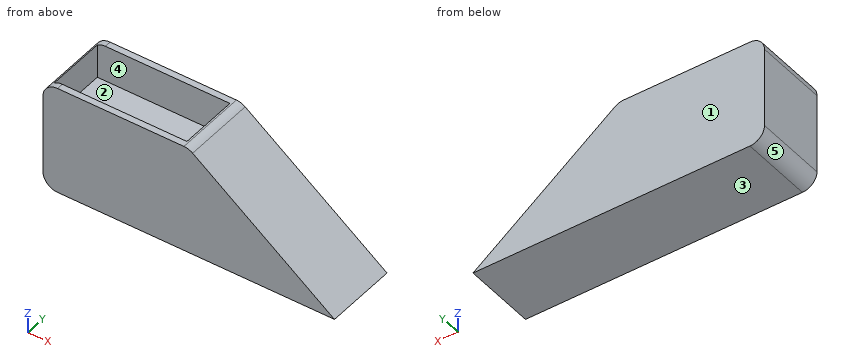
```python
from build123d import *

# Parameters (mm, degrees)
F1_DEPTH    = 25.4
F2_W        = 46.228
F2_H        = 20.828
F3_DEPTH    = 12.7
F4_T1_DEPTH = 50.8
F4_T3_DEPTH = 33.8666666667


# Not quite as in the source:
# - a fillet or chamfer that OpenCascade refuses, or shapes differently, is made with other operations: its cross-section is extruded or revolved along the edge and cut away or added


with BuildPart() as f1:
    # F0 (on Front) → F1 (new body)
    with BuildSketch(Plane.XZ):
        Polygon((0, 38.1), (0, 0), (101.6, 0), (50.8, 38.1), align=None)
    extrude(amount=F1_DEPTH)

    # F2 (on face) → F3 (cut)
    with BuildSketch(Plane.XY.offset(38.1)):
        with Locations((25.4, -12.7)):
            Rectangle(F2_W, F2_H)
    extrude(amount=-F3_DEPTH, mode=Mode.SUBTRACT)

    # F4: fillet of radius 5.08 on 3 edges, made by hand

    # F4_s2 → F4_t1 (cut)
    with BuildSketch(Plane.XZ.offset(-12.7)):
        with BuildLine():
            ThreePointArc((0, 33.02), (1.4878975516, 36.6121024484), (5.08, 38.1))
            Line((5.08, 38.1), (0, 38.1))
            Line((0, 38.1), (0, 33.02))
        make_face()
        with BuildLine():
            ThreePointArc((0, 5.08), (1.4878975516, 1.4878975516), (5.08, 0))
            Line((5.08, 0), (0, 0))
            Line((0, 0), (0, 5.08))
        make_face()
    extrude(amount=F4_T1_DEPTH, mode=Mode.SUBTRACT)

    # F4_s4 → F4_t3 (cut)
    with BuildSketch(Plane.XZ.offset(-4.2333333333)):
        with BuildLine():
            ThreePointArc((49.1066666667, 38.1), (50.713103718, 37.8393111541), (52.1546666667, 37.084))
            Line((52.1546666667, 37.084), (50.8, 38.1))
            Line((50.8, 38.1), (49.1066666667, 38.1))
        make_face()
    extrude(amount=F4_T3_DEPTH, mode=Mode.SUBTRACT)


solid = f1.part
```
Geometry check sheet. Reference: the model listing, model coordinates, mm. Face numbers are marked on the shaded views. A direction names the side the tool comes from. Round coordinates to 2 decimals unless told otherwise and drop trailing zeros. Loops run counter-clockwise (first coordinate to the right, second up) from the corner with the lowest first, then second, coordinate; pieces in that order, holes last. Notation, with made-up numbers: (28.5, 20.5) - (62.5, 20.5) arc R8 cw to (62.5, 29.5) - close; hole circle Ø1 at (59, -28.5). An arc over 180 degrees is marked (long way). Write each question's results on one line, items separated by ' | '. Start each with the question number.
Q1. Release check for a two-part mould opening along X. For the marked faces 3, 4 and 5 record: +X half, -X half, draft (parallel to the pull), parting line (faces both ways), or undercut.
Q2. Cross-section at B-B on x = 25.5. Enter the section's corners in (y, z), and give its area (3 significant figures).
Q3. Thickness scan on line 1 (Y direction, x = 32, z = 26); line 2 (Z direction, x = 39, y = -19.75); line 3 (X direction, y = -12.75, z = 28). Record the ranges inside material, lowest first. Write a range as [from, to].
Q4. Gauge pin test, flat ends, axial feed: P1, Ø1.5, axis at x = 15.5, z = 22, coming from the +Y side; P2, Ø6, axis at y = -21, z = 18, coming from the +X side; P3, Ø6, axis at y = -9.5, z = 30, coming from the +X side; P4, Ø4, axis at x = 56.5, y = -16, coming from the +Z side (3 decimals). Record the tip position at first contact, or that the pin passes through.
Q5. Cross-section at D-D on z = 12. Enter the section's corners in (x, y).
Q6. Cross-section at A-A on y = -22. Enter the section's corners in (x, z), and give its area (3 significant figures).
Q7. Access from +Z, -Z, +X, -X, +Y, -Y to the whole of each face (thin tool, end or side, straight path). Record for the marked faces 1 and 2.
Q8. Cross-section at C-C on z = 34. Enter the section's corners in (x, y).
Answers below:
1) face 3: draft | face 4: undercut | face 5: -X half
2) outline: (-25.4, 0) - (0, 0) - (0, 38.1) - (-2.29, 38.1) - (-2.29, 25.4) - (-23.11, 25.4) - (-23.11, 38.1) - (-25.4, 38.1) - close | area: 703 mm²
3) line 1: y = [-25.4, -23.11], [-2.29, 0] | line 2: z = [0, 25.4] | line 3: x = [0, 2.29], [48.51, 64.27]
4) P1: stops at y = 0 | P2: stops at x = 81.6 | P3: stops at x = 65.6 | P4: stops at z = 35.325
5) outline: (0, -25.4) - (85.6, -25.4) - (85.6, 0) - (0, 0) - close
6) outline: (0, 5.08) arc R5.08 ccw to (5.08, 0) - (101.6, 0) - (52.15, 37.08) arc R5.08 ccw to (49.11, 38.1) - (48.51, 38.1) - (48.51, 25.4) - (2.29, 25.4) - (2.29, 37.26) arc R5.08 ccw to (0, 33.02) - close | area: 2,310 mm²
7) face 1: +Z, -Z, +X, -X, +Y | face 2: +Z
8) outline: (0.1, -25.4) - (56.27, -25.4) - (56.27, 0) - (0.1, 0) - close; hole (2.29, -23.11) - (48.51, -23.11) - (48.51, -2.29) - (2.29, -2.29) - close
